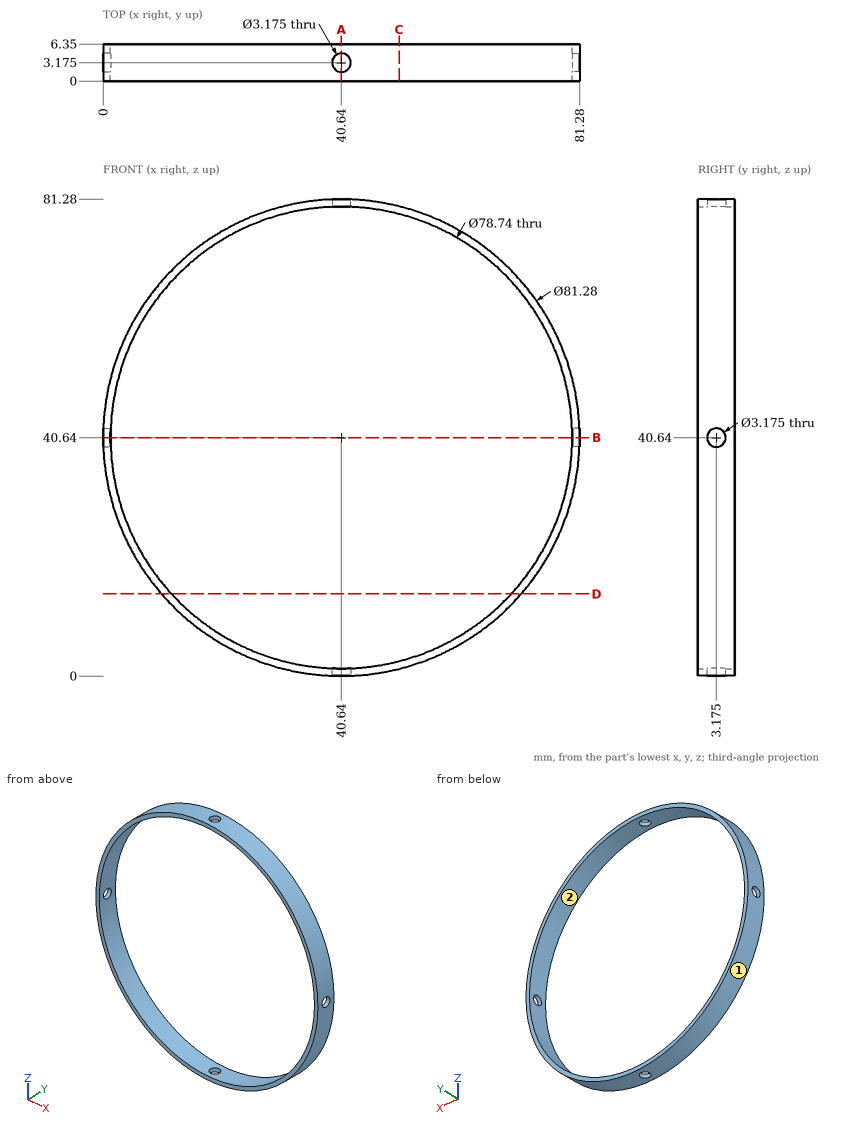
Study the drawing (mm; zero at the part's minimum x, y, z) and answer. Give positions to 0.01 mm unless a question says otherwise; leave off trailing zeros. Loops run counter-clockwise (first coordinate to the right, second up) from the corner with the lowest first, then second, coordinate; pieces in that order, holes last. Notation, with made-up numbers: M 40,18.5 L 76,18.5 A19 cw 76,40.5 Z; hole C 51,-7 d1. An arc over 180 degrees is marked long. One line per item, written item: value. Start each with the question number.
1. Each of these flat-tipped pins is pushed along its axis until it touches: P1, Ø3, axis at y = 3.175, z = 40.64, coming from the +X side; P2, Ø2, axis at y = 4.5, z = 71.5, coming from the +X side. Where does it stop, or does it pass through?
2. Find section D-D (z = 14). Give the vertices of the cut face in (x, y), and give its area (3 significant figures).
3. Find section B-B (z = 40.64). Give the vertices of the cut face in (x, y).
4. Find the intervals of material crossed by probe 1 along Z at (x, y) = (40.64, 5.25); probe 2 along Y at (x, z) = (40.64, 0.5); probe 3 along X at (y, z) = (1.25, 24), in increasing order.
5. Find section C-C (x = 50.5). Give the vertices of the cut face in (y, z), and give its area (3 significant figures).
6. Determine the mould class of the marked faces 1 and 2 for opening direction X: released by +X, released by -X, zero draft, split by the parting line, or undercut.
7. Find section A-A (x = 40.64). Give the vertices of the cut face in (y, z).
Reported:
1. P1: passes through
1. P2: stops at x = 68.21
2. outline: M 9.95,0 L 11.65,0 L 11.65,6.35 L 9.95,6.35 Z; M 69.63,0 L 71.33,0 L 71.33,6.35 L 69.63,6.35 Z
2. area: 21.6 mm²
3. outline: M 0,0 L 1.27,0 L 1.27,1.59 L 0,1.59 Z; M 0,4.76 L 1.27,4.76 L 1.27,6.35 L 0,6.35 Z; M 80.01,0 L 81.28,0 L 81.28,1.59 L 80.01,1.59 Z; M 80.01,4.76 L 81.28,4.76 L 81.28,6.35 L 80.01,6.35 Z
4. probe 1: z = 0 to 1.27, 80.01 to 81.28
4. probe 2: y = 0 to 1.59, 4.76 to 6.35
4. probe 3: x = 3.56 to 4.96, 76.32 to 77.72
5. outline: M 0,1.21 L 6.35,1.21 L 6.35,2.52 L 0,2.52 Z; M 0,78.76 L 6.35,78.76 L 6.35,80.07 L 0,80.07 Z
5. area: 16.6 mm²
6. face 1: split by the parting line
6. face 2: undercut
7. outline: M 0,0 L 1.59,0 L 1.59,1.27 L 0,1.27 Z; M 0,80.01 L 1.59,80.01 L 1.59,81.28 L 0,81.28 Z; M 4.76,0 L 6.35,0 L 6.35,1.27 L 4.76,1.27 Z; M 4.76,80.01 L 6.35,80.01 L 6.35,81.28 L 4.76,81.28 Z
